from build123d import *

# Parameters (mm, degrees)
F0_W            = 95
F0_H            = 50
F1_DEPTH        = 10
F2_R            = 10
F3_R            = 5
F4_DEPTH        = 10
F3_W            = 95
F3_H            = 25
F5_DEPTH        = 95
F6_W            = 40
F6_H            = 18
F7_DEPTH        = 95
F8_C1_SIZE2     = 20.9282884703
F8_C1_SIZE      = 57.5
F10_D           = 10
F10_CBORE_D     = 20
F10_CBORE_DEPTH = 10


with BuildPart() as f1:
    # F0 (on Front) → F1 (new body)
    with BuildSketch(Plane.XZ):
        Rectangle(F0_W, F0_H)
    extrude(amount=-F1_DEPTH)

    # F2
    f2_edges = [f1.edges().sort_by_distance(p)[0] for p in [
        (-47.5, 5, 25),
        (47.5, 5, 25),
    ]]
    fillet(f2_edges, radius=F2_R)

    # F3 (on face) → F4 (cut, through all)
    with BuildSketch(Plane.XZ):
        with Locations((-37.5, 15)):
            Circle(F3_R)
        with Locations((37.5, 15)):
            Circle(F3_R)
    extrude(amount=-F4_DEPTH, mode=Mode.SUBTRACT)

    # F3 (on face) → F5 (join)
    with BuildSketch(Plane.XZ):
        with Locations((0, -12.5)):
            Rectangle(F3_W, F3_H)
    extrude(amount=F5_DEPTH)

    # F6 (on face) → F7 (cut, through all)
    with BuildSketch(Plane.XZ.offset(95)):
        with Locations((0, -9)):
            Rectangle(F6_W, F6_H)
        with Locations((0, 9)):
            Rectangle(F6_W, F6_H)
    extrude(amount=-F7_DEPTH, mode=Mode.SUBTRACT)

    # F8: chamfer of 57.5 x 20.9282884703 on 2 edges, made by hand

    # F8_c1
    f8_c1_edges = [f1.edges().sort_by_distance(p)[0] for p in [
        (33.75, -95, 0),
    ]]
    f8_c1_side = f1.faces().sort_by_distance((33.75, -94.5814342306, 0))[0]
    chamfer(f8_c1_edges, length=F8_C1_SIZE, length2=F8_C1_SIZE2, reference=f8_c1_side)

    # F10 (through all)
    with Locations(Plane.XY):
        with Locations((-33.75, -18.75), (33.75, -18.75)):
            CounterBoreHole(F10_D / 2, F10_CBORE_D / 2, F10_CBORE_DEPTH)


solid = f1.part
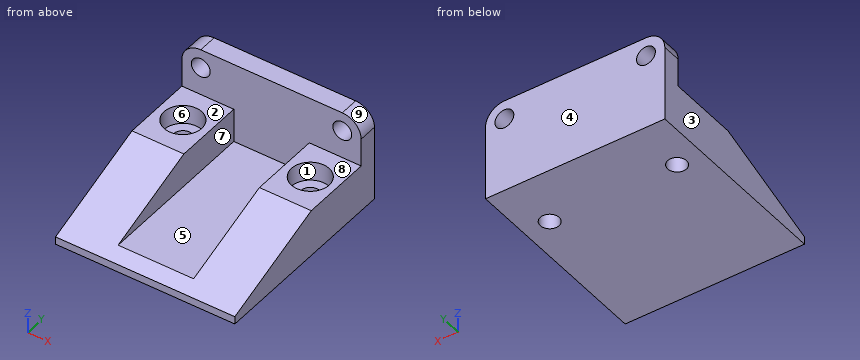
Model file for the job. Use its own axes, mm. Face numbers are marked on the shaded views. A direction names the side the tool comes from. Give positions to 0.01 mm unless a question says otherwise; leave off trailing zeros. Order: outer loops, then holes, each group sorted by start corner. A loop starts at its lowest first (then second) coordinate and runs counter-clockwise, first axis right, second up. Notation, with made-up numbers: M -23,12.5 L -7,12.5 A10 ccw -7,24.5 Z; hole C 15.25,42.5 d1. An arc over 180 degrees is marked long. Put each result on its own line as item: value. Start each with the question number.
(1) Band-saw the part on A-A on z = 12. Give the cut face in (x, y), then the cut area to 3 significant figures.
(2) Tool access for the marked faces 1, 2, 3, 4 and 5: list every direction of +Z, -Z, +X, -X, +Y, -Y with a clear straight run to the whole face (end or side of a thin tool).
(3) Band-saw the part on C-C on x = -33.75. Give the cut face in (y, z).
(4) Band-saw the part on D-D on x = -22.5. Give the cut face in (y, z).
(5) Band-saw the part on B-B on y = -18.75. Give the cut face in (x, z).
(6) Pull direction X, two halves, no side cores. Call the marked faces 6, 7, 8 and 9: released by +X, released by -X, zero draft, split by the parting line, or undercut.
(7) Drill centre lines: L1, parallel to Z at x = 37.5, y = 3.5; L2, parallel to X at y = -36, z = -9.5; L3, parallel to X at y = -18, z = -4. Where is each one in solid material? Low to high. Write a range as [from, to].
(8) Pin check, flat tips, straight feed: pin 1 Ø22 at (x, y) = (34.5, -19.5) entering from +Z; pin 2 Ø16 at (x, y) = (-33.75, -18.75) entering from +Z; pin 3 Ø5 at (x, y) = (19, -73.5) entering from +Z. Stop position of each tip, or through.
Results below:
1. outline: M -47.5,0 L -41.5,0 L -41.5,10 L -47.5,10 Z; M -33.5,0 L 33.5,0 L 33.5,10 L -33.5,10 Z; M 41.5,0 L 47.5,0 L 47.5,10 L 41.5,10 Z
1. area: 790 mm2
2. face 1: +Z
2. face 2: +Z, +X, -X, -Y
2. face 3: +Z, -Z, -X, +Y, -Y
2. face 4: +Z, -Z, +X, -X, +Y
2. face 5: +Z, -Y
3. outline: M -95,-25 L -23.75,-25 L -23.75,-10 L -28.75,-10 L -28.75,0 L -37.5,0 L -95,-20.93 Z; M -13.75,-25 L 10,-25 L 10,11.69 L 0,11.69 L 0,0 L -8.75,0 L -8.75,-10 L -13.75,-10 Z; M 0,18.31 L 10,18.31 L 10,25 L 0,25 Z
4. outline: M -95,-25 L 10,-25 L 10,25 L 0,25 L 0,0 L -37.5,0 L -95,-20.93 Z
5. outline: M -47.5,-25 L -38.75,-25 L -38.75,-10 L -43.75,-10 L -43.75,0 L -47.5,0 Z; M -28.75,-25 L 28.75,-25 L 28.75,-10 L 23.75,-10 L 23.75,0 L 20,0 L 20,-18 L -20,-18 L -20,0 L -23.75,0 L -23.75,-10 L -28.75,-10 Z; M 38.75,-25 L 47.5,-25 L 47.5,0 L 43.75,0 L 43.75,-10 L 38.75,-10 Z
6. face 6: undercut
6. face 7: undercut
6. face 8: zero draft
6. face 9: released by +X
7. L1: z = [-25, 10], [20, 25]
7. L2: x = [-47.5, -20], [20, 47.5]
7. L3: x = [-47.5, -43.72], [-23.78, -20], [20, 23.78], [43.72, 47.5]
8. pin 1: stops at z = 0
8. pin 2: stops at z = -10
8. pin 3: stops at z = -12.27
